from build123d import *

# Parameters (mm, degrees)
F0_W      = 100
F0_H      = 80
F1_DEPTH  = 45
F2_R      = 70
F3_DEPTH  = 20
F4_W      = 20
F4_H      = 15
F5_DEPTH  = 10
F7_DEPTH  = 25
F8_R      = 7.5
F9_DEPTH  = 30
F11_DEPTH = 80


with BuildPart() as f1:
    # F0 (on Top) → F1 (new body)
    with BuildSketch(Plane.XY):
        with Locations((50, 40)):
            Rectangle(F0_W, F0_H)
    extrude(amount=F1_DEPTH)

    # F2 (on face) → F3 (cut)
    with BuildSketch(Plane.XY.offset(45)):
        with Locations((0, -2.1579118226)):
            Circle(F2_R)
    extrude(amount=-F3_DEPTH, mode=Mode.SUBTRACT)

    # F4 (on face) → F5 (join)
    with BuildSketch(Plane.XY.offset(25)):
        with Locations((10, 7.5)):
            Rectangle(F4_W, F4_H)
    extrude(amount=F5_DEPTH)

    # F6 (on face) → F7 (cut, through all)
    with BuildSketch(Plane.XY.offset(25)):
        with BuildLine():
            ThreePointArc((62.176110422, 30), (50.6295075267, 46.1810265977), (35, 58.4638664423))
            Line((35, 58.4638664423), (35, 30))
            Line((35, 30), (62.176110422, 30))
        make_face()
    extrude(amount=-F7_DEPTH, mode=Mode.SUBTRACT)

    # F8 (on face) → F9 (cut)
    with BuildSketch(Plane.XY.offset(45)):
        with Locations((60, 65)):
            Circle(F8_R)
    extrude(amount=-F9_DEPTH, mode=Mode.SUBTRACT)

    # F10 (on face) → F11 (cut, through all)
    with BuildSketch(Plane.XZ):
        with BuildLine():
            ThreePointArc((83.6190264738, 45), (95.7773967757, 23.944395449), (100, 0))
            Line((100, 0), (100, 45))
            Line((100, 45), (83.6190264738, 45))
        make_face()
    extrude(amount=-F11_DEPTH, mode=Mode.SUBTRACT)


solid = f1.part
Geometry check sheet. Reference: the model listing, model coordinates, mm. A direction names the side the tool comes from. Round coordinates to 2 decimals unless told otherwise and drop trailing zeros. Write each loop counter-clockwise with the first axis right and the second up, starting at its lowest first coordinate (ties: lowest second). Pieces come first, ordered by that corner, then holes.
Item 1: Go/stop test with flat-tipped pins: pin 1 Ø2 at (x, y) = (23.5, 19.5) entering from +Z; pin 2 Ø8 at (y, z) = (29.5, 32) entering from -X; pin 3 Ø12 at (y, z) = (25.5, 17) entering from +X. Record where each tip stops, or that it passes through.
Determined:
pin 1: stops at z = 25
pin 2: stops at x = 60.24
pin 3: stops at x = 99.13
Item 2: Access from +Z, -Z, +X, -X, +Y, -Y to the whole of each face (thin tool, end or side, straight path). Record for faces 1 (the face through (10, 15, 30)), 2 (the face through (60, 65, 15)), 3 (the face through (10, 8, 35)), 4 (the face through (49, 0, 17)), 5 (the face through (48, 30, 13)).
Determined:
face 1: +Z, -X
face 2: +Z
face 3: +Z, -X, -Y
face 4: +Z, -Z, +X, -X, -Y
face 5: +Z, -Z
Item 3: Mould release check, pull along Y, two halves, no side actions. Record for faces 6 (the face through (54.5, 70.1, 30.2)), 7 (the face through (20, 7, 30)), 8 (the face through (49, 80, 22)): +Y half, -Y half, draft (parallel to the pull), parting line (faces both ways), or undercut.
Determined:
face 6: undercut
face 7: draft
face 8: +Y half
Item 4: Section check B-B (y = 41.5). Record the boundary of the cut face in (x, z).
Determined:
outline: (0, 0) - (35, 0) - (35, 25) - (0, 25) - close; (54.72, 0) - (100, 0) arc R70 ccw to (83.62, 45) - (54.72, 45) - close
Item 5: Section check C-C (x = 43). Record the boundary of the cut face in (y, z).
Determined:
outline: (0, 0) - (30, 0) - (30, 25) - (0, 25) - close; (53.08, 0) - (80, 0) - (80, 45) - (53.08, 45) - close
Item 6: Section check A-A (z = 29). Record the boundary of the cut face in (x, y).
Determined:
outline: (0, 0) - (20, 0) - (20, 15) - (0, 15) - close; (0, 67.84) arc R70 cw to (69.97, 0) - (93.71, 0) - (93.71, 80) - (0, 80) - close; hole circle Ø15 at (60, 65)
Item 7: Section check D-D (y = 11). Record the boundary of the cut face in (x, z).
Determined:
outline: (0, 0) - (100, 0) arc R70 ccw to (83.62, 45) - (68.75, 45) - (68.75, 25) - (20, 25) - (20, 35) - (0, 35) - close
Item 8: Material ranges on line 1 along Y through (x, z) = (60, 21); line 2 along Z through (x, y) = (42, 27.5); line 3 along X through (y, z) = (61.5, 33), recorded low to high.
Determined:
line 1: y = 0 to 30, 33.9 to 57.5, 72.5 to 80
line 2: z = 0 to 25
line 3: x = 29.11 to 53.37, 66.63 to 91.73
